Can you work these out from the model? Positions are in its coordinate system, mm. Coordinates: 2 decimals unless noted, no trailing zeros. Order: outer loops, then holes, each group sorted by start corner. A loop starts at its lowest first (then second) coordinate and runs counter-clockwise, first axis right, second up.
```python
from build123d import *

# Parameters (mm, degrees)
SKETCH1_W                 = 67.008250425
SKETCH1_H                 = 70
BOSS_EXTRUDE1_DEPTH       = 1.5
BOSS_EXTRUDE2_START       = -9.75
BOSS_EXTRUDE2_DEPTH       = 70
CUT_EXTRUDE1_START        = -6
CUT_EXTRUDE1_OUTLINE_W    = 73
CUT_EXTRUDE1_OUTLINE_H    = 4
CUT_EXTRUDE1_DEPTH        = 1.741494861
SKETCH4_W                 = 8
SKETCH4_H                 = 4.5
SKETCH4_W_2               = 5
SKETCH4_H_2               = 1.5
BOSS_EXTRUDE3_DEPTH       = 3
MIRROR2_COPY_1_SKETCH_W   = 8
MIRROR2_COPY_1_SKETCH_H   = 4.5
MIRROR2_COPY_1_SKETCH_W_2 = 5
MIRROR2_COPY_1_SKETCH_H_2 = 1.5
MIRROR2_COPY_1_DEPTH      = 3


with BuildPart() as part:
    # Sketch1 → Boss-Extrude1 (new body)
    with BuildSketch(Plane.XY):
        with Locations((29.175646202, 25.25)):
            Rectangle(SKETCH1_W, SKETCH1_H)
    extrude(amount=BOSS_EXTRUDE1_DEPTH)

    # Boss-Extrude2: read off the stored shape, not the designer's step
    # Boss-Extrude2 outline → Boss-Extrude2 (add)
    with BuildSketch(Plane(origin=(0, 0, 0), x_dir=(1, 0, 0), z_dir=(0, 1, 0)).offset(BOSS_EXTRUDE2_START)):
        Polygon((62.952808957, -1.5), (62.679771414, 0), (62.679771414, -1.5), align=None)
    extrude(amount=BOSS_EXTRUDE2_DEPTH)

    # Cut-Extrude1: read off the stored shape, not the designer's step
    # Cut-Extrude1 outline → Cut-Extrude1 (cut)
    with BuildSketch(Plane(origin=(0, 0, 0), x_dir=(0, 1, 0), z_dir=(0.9838340738940914, 0, -0.17908242528220206)).offset(CUT_EXTRUDE1_START)):
        with Locations((25.5, 0)):
            Rectangle(CUT_EXTRUDE1_OUTLINE_W, CUT_EXTRUDE1_OUTLINE_H)
    extrude(amount=CUT_EXTRUDE1_DEPTH, mode=Mode.SUBTRACT)

    # Sketch4 → Boss-Extrude3 (add)
    with BuildSketch(Plane(origin=(0, 0, 0), x_dir=(-1, 0, 0), z_dir=(0, 0, -1))):
        with Locations((-1.171520989, 56.5)):
            Rectangle(SKETCH4_W, SKETCH4_H)
        with Locations((-1.171520989, 56.5)):
            Rectangle(SKETCH4_W_2, SKETCH4_H_2, mode=Mode.SUBTRACT)
    boss_extrude3 = extrude(amount=BOSS_EXTRUDE3_DEPTH)

    # Mirror1: Boss-Extrude3 across plane
    add(boss_extrude3.mirror(Plane(origin=(29.175646202, 0, 0), x_dir=(0, 0, 1), z_dir=(1, 0, 0))))

    # Mirror2: Boss-Extrude3 across plane
    add(boss_extrude3.mirror(Plane(origin=(0, 25.25, 0), x_dir=(0, 0, 1), z_dir=(0, -1, 0))))

    # Mirror2 copy 1 sketch → Mirror2 copy 1 (add)
    with BuildSketch(Plane(origin=(58.351292403, 50.5, 0), x_dir=(1, 0, 0), z_dir=(0, 0, -1))):
        with Locations((-1.171520989, 56.5)):
            Rectangle(MIRROR2_COPY_1_SKETCH_W, MIRROR2_COPY_1_SKETCH_H)
        with Locations((-1.171520989, 56.5)):
            Rectangle(MIRROR2_COPY_1_SKETCH_W_2, MIRROR2_COPY_1_SKETCH_H_2, mode=Mode.SUBTRACT)
    extrude(amount=MIRROR2_COPY_1_DEPTH)


solid = part.part
```
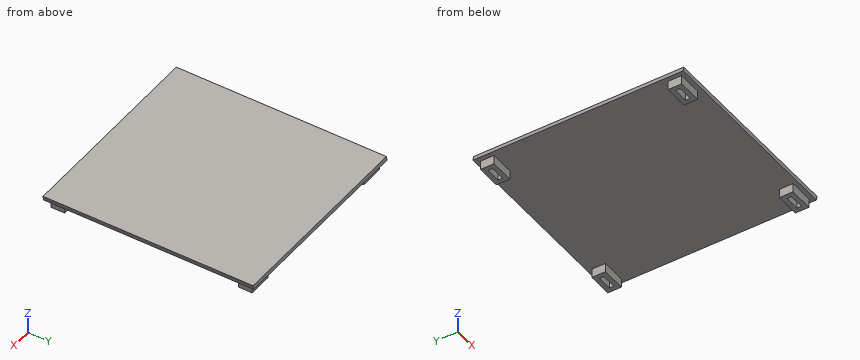
1. Imagine slicing it at A-A on z = -1.45. Give the number of separate pieces and of enclosed holes in the cut face, then the cut area to 3 significant figures.
Completed:
separate pieces: 4
enclosed holes: 4
area: 114 mm2
2. Please list where these lines run through material, in increasing order: probe 1 along X at (y, z) = (-6.5, -1.45); probe 2 along Y at (x, z) = (2.5, -2.05); probe 3 along X at (y, z) = (-4.5, -2.6).
Completed:
probe 1: x = -2.83 to -1.33, 3.67 to 5.17, 53.18 to 54.68, 59.68 to 61.18
probe 2: y = -8.25 to -6.75, -5.25 to -3.75, 54.25 to 55.75, 57.25 to 58.75
probe 3: x = -2.83 to 5.17, 53.18 to 61.18
3. I'm going to push flat-ended pins straight in: pin 1 (0.9 mm diameter, centred on y = 56, z = -1, fed in from -X); pin 2 (3 mm diameter, centred on x = 46.5, y = 29.5, fed in from -Z); pin 3 (2 mm diameter, centred on y = -1, z = -1.5, fed in from -X); pin 4 (2.5 mm diameter, centred on x = 1.5, z = -2, fed in from +Y). Where does each tip first touch, or does it pass through?
Completed:
pin 1: stops at x = -2.83
pin 2: stops at z = 0
pin 3: passes through
pin 4: stops at y = 58.75
4. Imagine slicing it at B-B on x = 1. Please give me the cut outline in (y, z), then the cut area to 3 significant figures.
Completed:
outline: (-9.75, 0) - (-8.25, 0) - (-8.25, -3) - (-6.75, -3) - (-6.75, 0) - (-5.25, 0) - (-5.25, -3) - (-3.75, -3) - (-3.75, 0) - (54.25, 0) - (54.25, -3) - (55.75, -3) - (55.75, 0) - (57.25, 0) - (57.25, -3) - (58.75, -3) - (58.75, 0) - (60.25, 0) - (60.25, 1.5) - (-9.75, 1.5) - close
area: 123 mm2
5. Imagine slicing it at C-C on y = 17. Please give me the cut outline in (x, z).
Completed:
outline: (-4.33, 0) - (62.68, 0) - (62.95, 1.5) - (-4.06, 1.5) - close
